Input: dimensioned drawing with shaded views. Units: mm. Origin: part minimum x, y, z. A direction names the side the tool comes from. Round coordinates to 2 decimals unless told otherwise and drop trailing zeros. Loops run counter-clockwise (first coordinate to the right, second up) from the corner with the lowest first, then second, coordinate; pieces in that order, holes last.
Item 1: Section query C-C on x = 6.5. Return loops of the section in (y, z), then the cut area to 3 significant figures.
Item 2: Pull-direction query (Z, two-part tool) for the marked faces 1, 2 and 3; classes: released by +Z, released by -Z, zero draft, split by the parting line, or undercut.
Item 3: Section query A-A on z = 6.25. Return loops of the section in (x, y) (1 decimal), then the cut area to 3 significant figures.
Item 4: Section query B-B on y = 12.5. Return loops of the section in (x, z).
Item 5: First-contact query: P1, Ø8, axis at y = 10.5, z = 12.5, coming from the -X side; P2, Ø2, axis at x = 10, y = 6.5, coming from the -Z side; P3, Ø3, axis at x = 18.5, z = 4.5, coming from the -Y side; P4, Ø1, axis at x = 27, z = 8, coming from the -Y side (1 decimal). Flat tips, straight axial feed; report the tip coordinate or a pass-through.
Item 6: Access query for the marked faces 4, 5 and 6. Directions: +Z, -Z, +X, -X, +Y, -Y. A direction counts if a zero-diameter tool reaches every point of the face in a straight line with its end or side. Return the directions, or none.
Item 7: Ray query, L1, parallel to Y at x = 3, z = 15; L2, parallel to X at y = 3, z = 8.25 (1 decimal); L3, parallel to Y at x = 29.5, z = 5.75 (1 decimal). Return the intervals inside material, ascending.
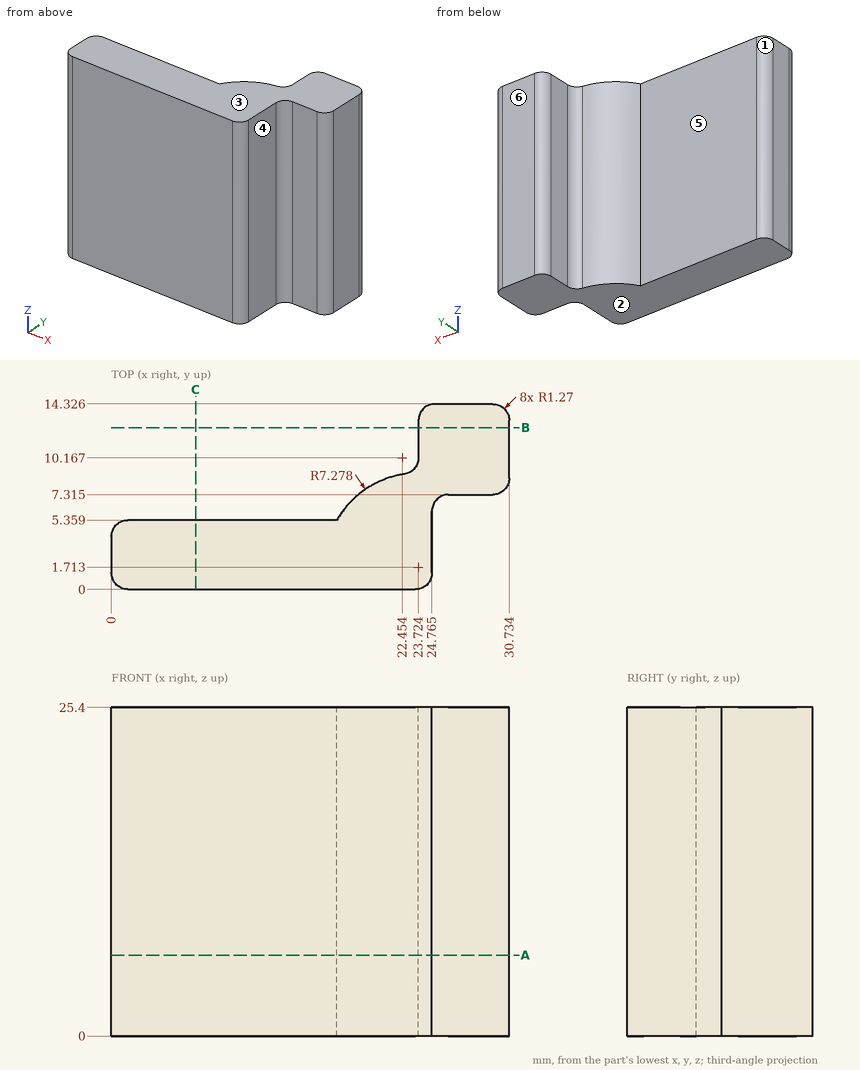
Data:
1. outline: (0, 0) - (5.36, 0) - (5.36, 25.4) - (0, 25.4) - close
1. area: 136 mm2
2. face 1: zero draft
2. face 2: released by -Z
2. face 3: released by +Z
3. outline: (0, 1.3) arc R1.3 ccw to (1.3, 0) - (23.5, 0) arc R1.3 ccw to (24.8, 1.3) - (24.8, 6) arc R1.3 cw to (26, 7.3) - (29.5, 7.3) arc R1.3 ccw to (30.7, 8.6) - (30.7, 13.1) arc R1.3 ccw to (29.5, 14.3) - (25, 14.3) arc R1.3 ccw to (23.7, 13.1) - (23.7, 10.2) arc R1.3 cw to (22.6, 8.9) arc R7.3 ccw to (17.4, 5.4) - (1.3, 5.4) arc R1.3 ccw to (0, 4.1) - close
3. area: 199 mm2
4. outline: (23.72, 0) - (30.73, 0) - (30.73, 25.4) - (23.72, 25.4) - close
5. P1: stops at x = 18.24
5. P2: passes through
5. P3: stops at y = 0
5. P4: stops at y = 7.3
6. face 4: +Z, -Z, +X, -Y
6. face 5: +Z, -Z, -X, +Y
6. face 6: +Z, -Z, +X, -X, +Y
7. L1: y = 0 to 5.36
7. L2: x = 0 to 24.8
7. L3: y = 7.3 to 14.3
